Design review of the part shown in the three views and the two pictorial views. Dimensions are in mm from the part's minimum x, y and z. Coordinates: 2 decimals unless noted, no trailing zeros. Answer as CSV lines item,"result". Start each with the question number.
Q1. Mouldability with a two-part tool opening along Z and no side actions: class the marked faces 1, 2 and 3 as pulls with the +Z half, pulls with the -Z half, needs draft (parallel to the pull), parting line crosses it, or undercut.
Q2. Clearance check with flat-ended pins moving along their axes: pin 1 (5.5 mm diameter, centred on y = 7.94, z = 7.94, fed in from -X); pin 2 (1 mm diameter, centred on x = 2.5, y = 11.5, fed in from +Z). State where each tip first meets the part, or that it passes through.
Q3. For line 1 along Z through (x, y) = (3.8, 7) (1 decimal); line 2 along Z through (x, y) = (4.05, 9.5) (1 decimal), list the stretches that pass through material, from the lowest coordinate up. Write a range as [from, to].
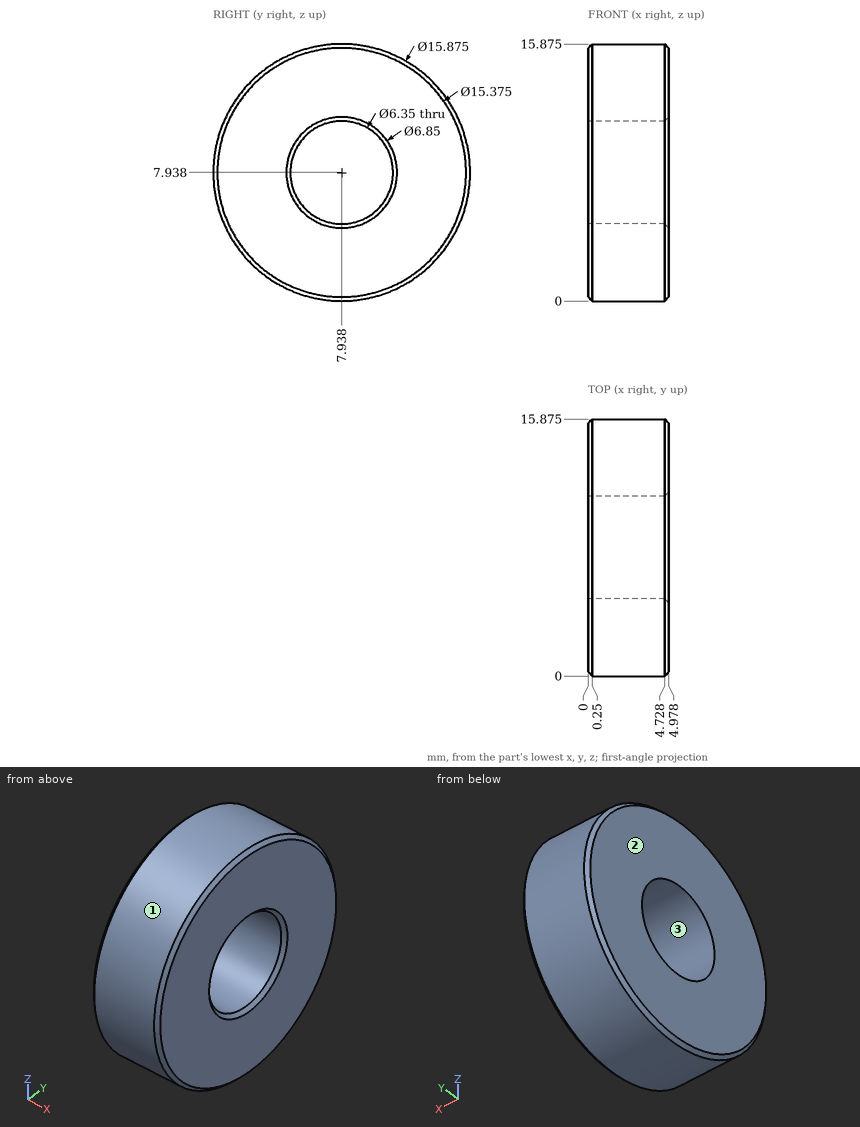
Results list:
1,face 1,"parting line crosses it"
1,face 2,"needs draft"
1,face 3,"undercut"
2,pin 1,"passes through"
2,pin 2,"stops at z = 15.26"
3,line 1,"z = [0.1, 4.9], [11, 15.8]"
3,line 2,"z = [0.2, 5.2], [10.7, 15.7]"
